Part print with two shaded views. Sizes in mm from the minimum x, y, z corner. Give positions to 0.01 mm unless a question says otherwise; leave off trailing zeros. Write each loop counter-clockwise with the first axis right and the second up, starting at its lowest first coordinate (ties: lowest second). Pieces come first, ordered by that corner, then holes. Notation, with made-up numbers: (-18, 79) - (-11, 79) arc R9 ccw to (-11, 95) - close; hole circle Ø1 at (23, 72). An arc over 180 degrees is marked (long way). One line per item, written item: value. Start each with the question number.
(1) Probe L1, parallel to Y at x = 9.2, z = 7.5; L2, parallel to X at y = 4.5, z = 3.5 (1 decimal); L3, parallel to X at y = 6.75, z = 11.5 (1 decimal). List the from-to ranges inside material, lowest first.
(2) Mould opens along Z. For the marked faces 1, 2 and 3 say: pulls with the +Z half, pulls with the -Z half, needs draft (parallel to the pull), parting line crosses it, or undercut.
(3) Cut at A-A, the plane x = 9.2. List the corners of the cut face in (y, z), and give its area (3 significant figures).
(4) Drop flat-ended pins along their axis: P1, Ø1, axis at y = 7, z = 1, coming from the -X side; P2, Ø6.5, axis at x = 9.5, z = 7, coming from the -Y side. Give the stop position or say it passes through.
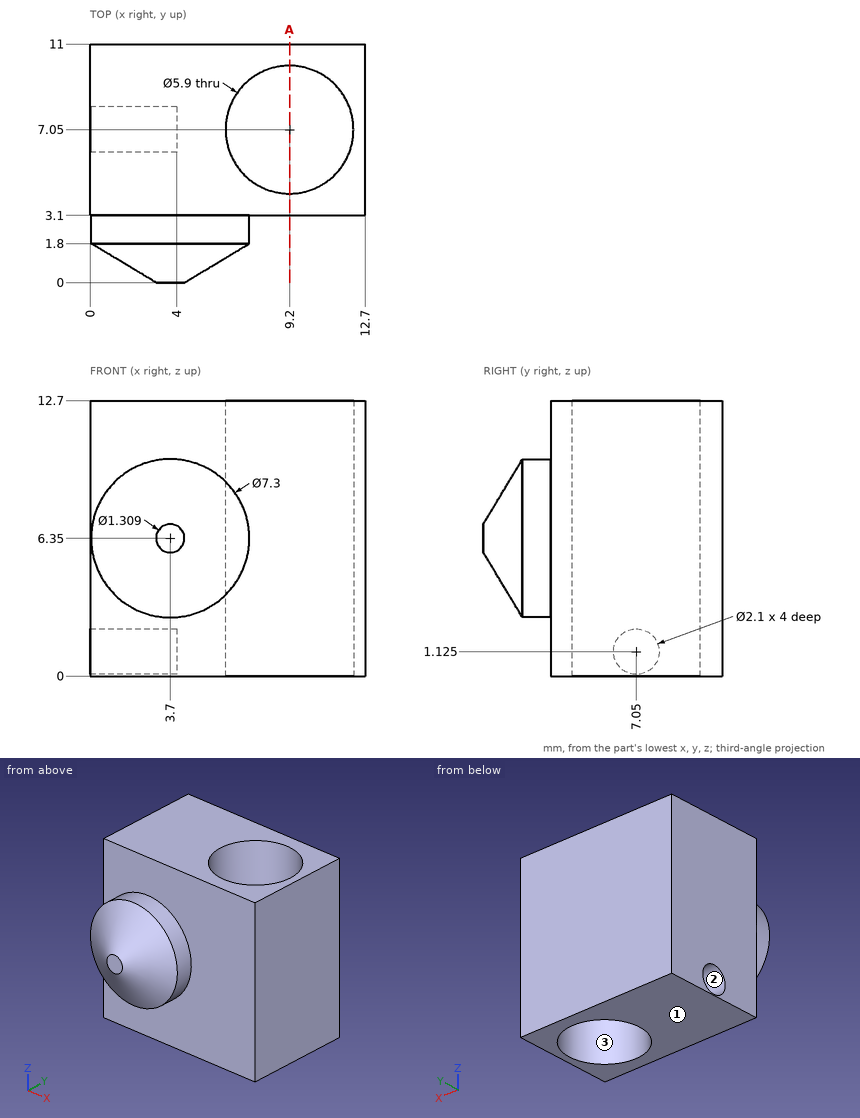
Answers follow:
1. L1: y = 3.1 to 4.1, 10 to 11
1. L2: x = 0 to 7.7, 10.7 to 12.7
1. L3: x = 0 to 6.3, 12.1 to 12.7
2. face 1: pulls with the -Z half
2. face 2: undercut
2. face 3: needs draft
3. outline: (3.1, 0) - (4.1, 0) - (4.1, 12.7) - (3.1, 12.7) - close; (10, 0) - (11, 0) - (11, 12.7) - (10, 12.7) - close
3. area: 25.4 mm²
4. P1: stops at x = 4
4. P2: stops at y = 1.16
